Autodesk Inventor part; units mm, degrees
ref_plane "YZ Plane" through (0, 0, 0) normal (1, 0, 0) x (0, 1, 0)
ref_plane "XZ Plane" through (0, 0, 0) normal (0, 1, 0) x (-1, 0, 0)
ref_plane "XY Plane" through (0, 0, 0) normal (0, 0, 1) x (1, 0, 0)
sketch "Skizze1" plane through (0, 0, 0) normal (0, 0, 1) x (1, 0, 0)
  line L0 (-45, -15) -> (45, -15)
  line L1 (45, -15) -> (45, 15)
  line L2 (45, 15) -> (-45, 15)
  line L3 (-45, 15) -> (-45, -15)
  line L4 (-45, -15) -> (45, 15) construction
  line L5 (45, -15) -> (-45, 15) construction
  circle A0 centre (-33.4649, 0) radius 1.5
  circle A1 centre (33.4649, 0) radius 1.5
  line L6 (0, -21) -> (0, 21) construction
  line L7 (-63, 0) -> (63, 0) construction
  line L8 (-5.25, 7) -> (5.25, 7)
  line L9 (5.25, 7) -> (5.25, -7)
  line L10 (5.25, -7) -> (-5.25, -7)
  line L11 (-5.25, -7) -> (-5.25, 7)
  circle A2 centre (-2.6, 3.85) radius 1.65 construction
  circle A3 centre (-2.6, 3.85) radius 1.25
  circle A4 centre (-2.6, 3.85) radius 2.5
  line L12 (-5.25, 1.35) -> (-2.6, 1.35)
  line L13 (-0.1, 3.85) -> (-0.1, 7)
  line L14 (-5.25, 1.35) -> (-5.25, 7)
  line L15 (-5.25, 7) -> (-0.1, 7)
  line L16 (-3.75, -15) -> (3.75, -15)
  line L17 (3.75, -15) -> (3.75, -7)
  line L18 (3.75, -7) -> (-3.75, -7)
  line L19 (-3.75, -7) -> (-3.75, -15)
  point P0 (0, 0)
  point P1 (0, -7)
  point P2 (-5.25, -15)
  point P3 (-5.25, -4.15)
  point P4 (5.25, 0)
  point P5 (0, -15)
  dimension "d0" = 66.9299
  dimension "d1" = 30
  dimension "d2" = 90
  dimension "d3" = 3
  dimension "d6" = 14
  dimension "d7" = 10.5
  dimension "d8" = 1
  dimension "d9" = 1.5
  dimension "d10" = 3.3
  dimension "d11" = 2.5
  dimension "d16" = 5
  dimension "d18" = 7.5
extrude "Extrusion2" add sketch "Skizze1" along normal blind 4 contours L3 L2 L1 L0 L17 L10 L9 L8 L11 L19 | L19 L10 L17 L0
extrude "Extrusion3" add sketch "Skizze1" along normal blind 1.5 contours L11 L8 L13 A4 L12 | A4
extrude "Extrusion6" cut sketch "Skizze1" along normal blind 2 contours L19 L10 L17 L0
fillet "Rundung1" radius 4 4 edges at (-45, -15, 2) (-45, 15, 2) (45, 15, 2) (45, -15, 2)
sketch "Skizze2" plane through (0, 0, 4) normal (0, 0, 1) x (1, 0, 0)
  circle A0 centre (-33.4649, 0) radius 1.5
  circle A1 centre (33.4649, 0) radius 1.5
  point P0 (0, 0)
  point P1 (32.8585, 1.3744)
hole "Bohrung1" at (-33.4649, 0, 4) at (33.4649, 0, 4) direction (0, 0, -1) diameter 3.4 end through all counterbore diameter 6.5 counterbore depth 3
extrude "Extrusion7" add sketch "Skizze1" along normal blind 2.5 contours A3
properties part number "BMP280_Holder"
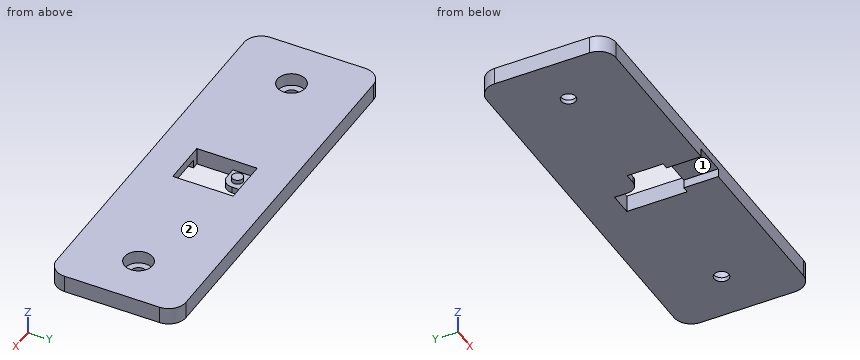
Model file for the job. Use its own axes, mm. Face numbers are marked on the shaded views. Round coordinates to 2 decimals unless told otherwise and drop trailing zeros. Loops run counter-clockwise (first coordinate to the right, second up) from the corner with the lowest first, then second, coordinate; pieces in that order, holes last. Notation, with made-up numbers: M -8,70 L 19,70 A14 ccw 19,81 Z; hole C 37,-8.5 d8. An arc over 180 degrees is marked long. Put each result on its own line as item: value. Start each with the question number.
Item 1: Cut at A-A (y = 0). List the corners of the cut face in (x, z), then the cut area to 3 significant figures.
Item 2: Drop flat-ended pins along their axis: P1, Ø2.5, axis at x = -3, y = 4.5, coming from the +Z side; P2, Ø4, axis at x = -33.46, y = 0, coming from the -Z side; P3, Ø4, axis at x = 0, y = -9.5, coming from the -Z side; P4, Ø2, axis at y = -13, z = 1, coming from the +X side. Give the stop position or say it passes through.
Item 3: Drill centre lines: line 1 along X through (y, z) = (0, 2.9); line 2 along X through (y, z) = (0, 0.7); line 3 along X through (y, z) = (-3.75, 2.65). Where is each one in solid material? Low to high.
Item 4: Cut at B-B (y = 6). List the corners of the cut face in (x, z), then the cut area to 3 significant figures.
Item 5: Mould opens along X. For the marked faces 1 and 2 say: released by +X, released by -X, zero draft, split by the parting line, or undercut.
Item 6: Cut at C-C (x = -31). List the corners of the cut face in (y, z), then the cut area to 3 significant figures.
Answer block:
1. outline: M -45,0 L -35.16,0 L -35.16,1 L -36.71,1 L -36.71,4 L -45,4 Z; M -31.76,0 L -5.25,0 L -5.25,4 L -30.21,4 L -30.21,1 L -31.76,1 Z; M 5.25,0 L 31.76,0 L 31.76,1 L 30.21,1 L 30.21,4 L 5.25,4 Z; M 35.16,0 L 45,0 L 45,4 L 36.71,4 L 36.71,1 L 35.16,1 Z
1. area: 272 mm2
2. P1: z = 2.5
2. P2: z = 0
2. P3: z = 2
2. P4: x = 44.87
3. line 1: -45 to -36.71, -30.21 to -5.25, 5.25 to 30.21, 36.71 to 45
3. line 2: -45 to -35.16, -31.76 to -5.25, 5.25 to 31.76, 35.16 to 45
3. line 3: -45 to -5.25, 5.25 to 45
4. outline: M -45,0 L -0.1,0 L -0.1,1.5 L -5.25,1.5 L -5.25,4 L -45,4 Z; M 5.25,0 L 45,0 L 45,4 L 5.25,4 Z
4. area: 326 mm2
5. face 1: undercut
5. face 2: zero draft
6. outline: M -15,0 L 15,0 L 15,4 L 2.12,4 L 2.12,1 L -2.12,1 L -2.12,4 L -15,4 Z
6. area: 107 mm2
